Can you work these out from the drawing? Everything is in mm from the part's minimum corner. A direction names the side the tool comes from. Round coordinates to 2 decimals unless told otherwise and drop trailing zeros. Write each loop counter-clockwise with the first axis right and the second up, starting at its lowest first coordinate (ties: lowest second). Pieces come first, ordered by that corner, then holes. Notation, with made-up numbers: (14, 9) -> (43, 9) arc R10 cw to (43, 14) -> close; hole circle Ø3 at (3, -15.5). An arc over 180 degrees is marked (long way). Write item = value, one per line. Start each with the question number.
1) Thinking about a two-plate mould opening in Y: for the marked faces 1, 2 and 3, which applies, +Y half, -Y half, draft (parallel to the pull), parting line (faces both ways), or undercut?
2) Imagine slicing it at A-A, the plane x = 9.8. Please give me the cut outline in (y, z).
3) I'm going to push flat-ended pins straight in: pin 1 (1 mm diameter, centred on y = 21.5, z = 1.5, fed in from -X); pin 2 (1 mm diameter, centred on x = 12.5, z = 2, fed in from +Y); pin 3 (2 mm diameter, centred on x = 1.5, z = 2.5, fed in from -Y). Where does each tip first touch, or does it pass through?
4) Imagine slicing it at C-C, the plane y = 22. Please give me the cut outline in (x, z).
5) Imagine slicing it at B-B, the plane z = 2.6. State how many separate pieces and enclosed holes the cut face has.
6) For the marked faces 4, 5 and 6, which set-ups out of +Z, -Z, +X, -X, +Y, -Y let a thin tool reach every point of the face, with its end or its side?
7) Imagine slicing it at D-D, the plane y = 2. Please give me the cut outline in (x, z).
8) If I drill on line 1 (Y direction, x = 10.75, z = 3.1); line 2 (X direction, y = 1.75, z = 0.85); line 3 (X direction, y = 12.25, z = 0.4), over which ranges is the centre line in solid material (lowest first)?
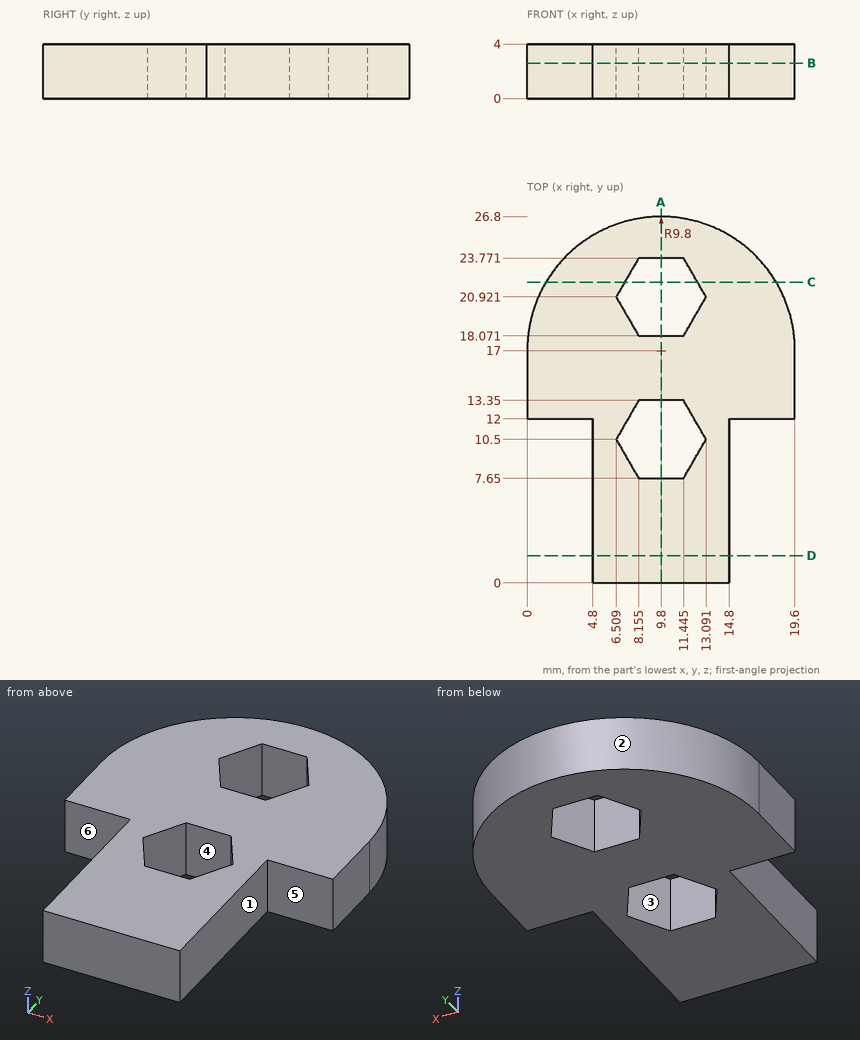
Reported:
q1.face_1 = draft
q1.face_2 = +Y half
q1.face_3 = undercut
q2.outline = (0, 0) -> (7.65, 0) -> (7.65, 4) -> (0, 4) -> close; (13.35, 0) -> (18.07, 0) -> (18.07, 4) -> (13.35, 4) -> close; (23.77, 0) -> (26.8, 0) -> (26.8, 4) -> (23.77, 4) -> close
q3.pin_1 = 0.85
q3.pin_2 = 26.55
q3.pin_3 = 12
q4.outline = (1.37, 0) -> (7.13, 0) -> (7.13, 4) -> (1.37, 4) -> close; (12.47, 0) -> (18.23, 0) -> (18.23, 4) -> (12.47, 4) -> close
q5.separate_pieces = 1
q5.enclosed_holes = 2
q6.face_4 = +Z, -Z
q6.face_5 = +Z, -Z, +X, -Y
q6.face_6 = +Z, -Z, -X, -Y
q7.outline = (4.8, 0) -> (14.8, 0) -> (14.8, 4) -> (4.8, 4) -> close
q8.line_1 = 0 to 7.65, 13.35 to 18.07, 23.77 to 26.75
q8.line_2 = 4.8 to 14.8
q8.line_3 = 0 to 7.52, 12.08 to 19.6
